Work out the finished part from the listing and answer in its coordinate system (mm). A direction names the side the tool comes from. Give positions to 0.01 mm unless a question says otherwise; leave off trailing zeros. Loops run counter-clockwise (first coordinate to the right, second up) from the corner with the lowest first, then second, coordinate; pieces in that order, holes last.
from build123d import *

# Parameters (mm, degrees)
F0_R     = 6.35
F0_R_2   = 2.54
F1_DEPTH = 7.874
F2_R     = 2.54
F3_DEPTH = 11.43
F4_R     = 2.54
F5_DEPTH = 3.556


with BuildPart() as f1:
    # F0 (on Top) → F1 (new body)
    with BuildSketch(Plane.XY):
        Circle(F0_R)
        Circle(F0_R_2, mode=Mode.SUBTRACT)
    extrude(amount=F1_DEPTH)

    # F2 (on Top) → F3 (join)
    with BuildSketch(Plane.XY):
        Circle(F2_R)
    extrude(amount=F3_DEPTH)

    # F4 (on Top) → F5 (join)
    with BuildSketch(Plane.XY):
        Circle(F4_R)
    extrude(amount=-F5_DEPTH)


solid = f1.part
Item 1: Consider line 1 (Z direction, x = -2, y = 2); line 2 (Y direction, x = 0, z = 10.75); line 3 (Y direction, x = -0.25, z = 6). Determine where each line is inside the solid, lowest interval first.
Item 2: Find section A-A, the plane y = 0. Write down the section's boundary in (x, z).
Item 3: For faces 1 (the face through (3, 0, 0)), 2 (the face through (3, 0, 7.874)), 3 (the face through (0, 0, -3.556)), determine the directions among +Z, -Z, +X, -X, +Y, -Y from which every point of the face is accessible in a straight line to the end or side of a thin tool.
Item 4: Flat-ended cylindrical pins translate along their axes: pin 1 Ø4 at (y, z) = (4.5, 2) entering from +X; pin 2 Ø2 at (y, z) = (2.5, 7) entering from -X; pin 3 Ø4 at (x, z) = (-5, -1.5) entering from -Y; pin 4 Ø1 at (x, z) = (3.5, -1.5) entering from +Y. Find the tip coordinate at first contact, or state that the pin passes through.
Item 5: Find section D-D, the plane z = 9.25. Write down the section's boundary in (x, y), plus the area to 3 significant figures.
Item 6: Find section C-C, the plane z = 2.5. Write down the section's boundary in (x, y).
Ans:
1. line 1: z = 0 to 7.87
1. line 2: y = -2.54 to 2.54
1. line 3: y = -6.35 to 6.35
2. outline: (-6.35, 0) - (-2.54, 0) - (-2.54, -3.56) - (2.54, -3.56) - (2.54, 0) - (6.35, 0) - (6.35, 7.87) - (2.54, 7.87) - (2.54, 11.43) - (-2.54, 11.43) - (-2.54, 7.87) - (-6.35, 7.87) - close
3. face 1: -Z
3. face 2: +Z
3. face 3: -Z, +X, -X, +Y, -Y
4. pin 1: stops at x = 5.84
4. pin 2: stops at x = -6.17
4. pin 3: stops at y = -5.18
4. pin 4: passes through
5. outline: circle Ø5.08 at (0, 0)
5. area: 20.3 mm2
6. outline: circle Ø12.7 at (0, 0)
